from build123d import *

# Parameters (mm, degrees)
RESSALTO_EXTRUS_O1_DEPTH  = 3
ESBO_O2_W                 = 47.384173958
ESBO_O2_H                 = 2
RESSALTO_EXTRUS_O2_DEPTH  = 3
RESSALTO_EXTRUS_O3_DEPTH  = 2
RESSALTO_EXTRUS_O5_DEPTH  = 12
CORTE_EXTRUS_O1_DEPTH     = 131
CORTE_EXTRUS_O3_DEPTH     = 10
RESSALTO_EXTRUS_O13_DEPTH = 120.5
RESSALTO_EXTRUS_O14_DEPTH = 10
ESBO_O20_W                = 100.5
ESBO_O20_H                = 2
CORTE_EXTRUS_O6_DEPTH     = 150.3


with BuildPart() as part:
    # Esboço1 → Ressalto-extrusão1 (new body)
    with BuildSketch(Plane(origin=(0, 0, 0), x_dir=(1, 0, 0), z_dir=(0, 1, 0))):
        Polygon((53.693575035, 0), (26.846787517, 46.5), (-26.846787517, 46.5), (-53.693575035, 0), (-26.846787517, -46.5), (26.846787517, -46.5), align=None)
    extrude(amount=RESSALTO_EXTRUS_O1_DEPTH)

    # Esboço2 → Ressalto-extrusão2 (add)
    with BuildSketch(Plane(origin=(0, 3, 0), x_dir=(1, 0, 0), z_dir=(0, 1, 0))):
        with Locations((0, 43.5)):
            Rectangle(ESBO_O2_W, ESBO_O2_H)
        Polygon((-50.384173958, -1.732050808), (-26.692086979, -42.767949192), (-24.960036171, -41.767949192), (-48.65212315, -0.732050808), align=None)
        Polygon((26.692086979, -42.767949192), (50.384173958, -1.732050808), (48.65212315, -0.732050808), (24.960036171, -41.767949192), align=None)
    extrude(amount=RESSALTO_EXTRUS_O2_DEPTH)

    # Esboço3 → Ressalto-extrusão3 (add)
    with BuildSketch(Plane.XZ):
        Polygon((26.846787517, 46.5), (-26.846787517, 46.5), (-53.693575035, 0), (-26.846787517, -46.5), (26.846787517, -46.5), (53.693575035, 0), align=None)
    extrude(amount=RESSALTO_EXTRUS_O3_DEPTH)

    # Esboço5 → Ressalto-extrusão5 (add)
    with BuildSketch(Plane.XZ.offset(2)):
        with BuildLine():
            Line((38, 49.00146682), (38, -77.5))
            ThreePointArc((38, -77.5), (36.828427125, -80.328427125), (34, -81.5))
            Line((34, -81.5), (-34, -81.5))
            ThreePointArc((-34, -81.5), (-36.828427125, -80.328427125), (-38, -77.5))
            Line((-38, -77.5), (-38, 49.00146682))
            ThreePointArc((-38, 49.00146682), (-36.828427125, 51.829893945), (-34, 53.00146682))
            Line((-34, 53.00146682), (34, 53.00146682))
            ThreePointArc((34, 53.00146682), (36.828427125, 51.829893945), (38, 49.00146682))
        make_face()
    extrude(amount=RESSALTO_EXTRUS_O5_DEPTH)

    # Esboço7 → Corte-extrusão1 (cut)
    with BuildSketch(Plane(origin=(0, 0, -81.5), x_dir=(-1, 0, 0), z_dir=(0, 0, -1))):
        Polygon((-34.2, -3), (34.2, -3), (34.2, -12.3), (31.2, -12.3), (31.2, -23.281359025), (-31.2, -26.250413902), (-31.2, -12.3), (-34.2, -12.3), align=None)
    extrude(amount=-CORTE_EXTRUS_O1_DEPTH, mode=Mode.SUBTRACT)

    # Esboço8 → Corte-extrusão3 (cut)
    with BuildSketch(Plane.XZ.offset(2)):
        Polygon((-48.693575035, 0), (-38, 0), (-38, -18.521815275), align=None)
        Polygon((38, 0), (48.693575035, 0), (38, -18.521815275), align=None)
    extrude(amount=-CORTE_EXTRUS_O3_DEPTH, mode=Mode.SUBTRACT)

    # Esboço17 → Ressalto-extrusão13 (add)
    with BuildSketch(Plane(origin=(0, 0, -71.5), x_dir=(-1, 0, 0), z_dir=(0, 0, -1))):
        Polygon((-53.25, -20), (-53.25, -18), (-53.25, -10), (-38, -2), (-38, -6), (-38, -10), (-48.25, -12.68852459), (-48.25, -18), (-48.25, -20), (-48.25, -22), (-48.25, -24), (-53.25, -24), (-53.25, -22), align=None)
        Polygon((53.25, -20), (53.25, -18), (53.25, -10), (38, -2), (38, -6), (38, -10), (48.25, -12.68852459), (48.25, -18), (48.25, -20), (48.25, -22), (48.25, -24), (53.25, -24), align=None)
    extrude(amount=-RESSALTO_EXTRUS_O13_DEPTH)

    # Esboço19 → Ressalto-extrusão14 (add, symmetric)
    with BuildSketch(Plane(origin=(0, 0, 0), x_dir=(0, 0, -1), z_dir=(1, 0, 0))):
        Polygon((-53.00146682, -14), (-53.00146682, -2), (-82, -10), (-82, -24), (-76, -24), (-76, -18), align=None)
    extrude(amount=RESSALTO_EXTRUS_O14_DEPTH, both=True)

    # Esboço20 → Corte-extrusão6 (cut)
    with BuildSketch(Plane(origin=(0, 0, -71.5), x_dir=(-1, 0, 0), z_dir=(0, 0, -1))):
        with Locations((0, -21)):
            Rectangle(ESBO_O20_W, ESBO_O20_H)
    extrude(amount=-CORTE_EXTRUS_O6_DEPTH, mode=Mode.SUBTRACT)


solid = part.part
Could you check a few things on this model? Use its own coordinates, in mm. A direction names the side the tool comes from. Coordinates: 2 decimals unless noted, no trailing zeros. Write each loop counter-clockwise with the first axis right and the second up, starting at its lowest first coordinate (ties: lowest second). Pieces come first, ordered by that corner, then holes. Notation, with made-up numbers: M 22,-36.75 L 29,-36.75 A22 ccw 29,-12.75 Z; hole C -8.5,-8.5 d9. An arc over 180 degrees is marked long. One line per question, with ' | ' between items.
1) For pin 1 Ø5 at (x, y) = (-15.5, 2.5) entering from +Z; pin 2 Ø10 at (y, z) = (-13.5, 12.5) entering from +X; pin 3 Ø5 at (y, z) = (-7.5, 65.5) entering from +X, each with a flat end and sliding along its axis, tell me the tip position at first contact or that it passes through.
Checks:
pin 1: z = 46.5 | pin 2: x = 53.25 | pin 3: x = 10
2) If we mould it in two halves opening along Z, with no side actions, what happens to faces 6 (the face through (-38, 1, -9)), 7 (the face through (-34.2, -8, -17)), 8 (the face through (-43, 0, 0)), 9 (the face through (0.14, -16.028, 64.662))? For each: released by +Z, released by -Z, zero draft, split by the parting line, or undercut.
Checks:
face 6: undercut | face 7: zero draft | face 8: undercut | face 9: released by -Z
3) Imagine slicing it at D-D, the plane x = 46. Write out the boundary of the cut face in (y, z), and give its area (3 significant figures).
Checks:
outline: M -12.1,-71.5 L -6.2,-71.5 L -6.2,49 L -12.1,49 Z; M -2,-13.33 L 3,-13.33 L 3,-4.67 L -2,-4.67 Z; M -2,0 L 3,0 L 3,5.33 L 6,5.33 L 6,9.33 L 3,9.33 L 3,13.33 L -2,13.33 Z | area: 833 mm²
4) I need wall thicknesses on probe 1 along X at (y, z) = (-21.5, -52.5); probe 2 along Y at (x, z) = (-32, -71); probe 3 along X at (y, z) = (-11.5, -74). Which ranges of each line are inside material? Lowest first, please. Write a range as [from, to].
Checks:
probe 1: [-53.25, -50.25], [50.25, 53.25] | probe 2: [-14, -12.3], [-3, -2] | probe 3: [-38, -34.2], [34.2, 38]
5) Imagine slicing it at C-C, the plane x = 13.5. Write out the boundary of the cut face in (y, z).
Checks:
outline: M -14,49.5 L -3,49.5 L -3,-81.5 L -2,-81.5 L -2,-46.5 L 3,-46.5 L 3,-44.5 L 6,-44.5 L 6,-42.5 L 3,-42.5 L 3,46.5 L -2,46.5 L -2,53 L -14,53 Z
6) For faces 1 (the face through (-36.64, 4.48, 21.54)), 2 (the face through (40.46, 0.54, 22.92)), 3 (the face through (34.2, -8, -17)), 4 (the face through (47, -10, 49)), 5 (the face through (-48.25, -16, -12)), which set-ups out of +Z, -Z, +X, -X, +Y, -Y let a thin tool reach every point of the face, with its end or its side?
Checks:
face 1: -Z, +Y | face 2: +Z, +X, +Y | face 3: -Z | face 4: +Z, +X, +Y, -Y | face 5: +Z, -Z, -Y
7) Imagine slicing it at A-A, the plane y = 0.5. Write out the boundary of the cut face in (x, z).
Checks:
outline: M -53.69,0 L -26.85,-46.5 L 26.85,-46.5 L 53.69,0 L 26.85,46.5 L -26.85,46.5 Z; hole M -48.69,0 L -38,-18.52 L -38,0 Z; hole M 38,-18.52 L 48.69,0 L 38,0 Z
